Could you check a few things on this model? Use its own coordinates, in mm. A direction names the side the tool comes from. Coordinates: 2 decimals unless noted, no trailing zeros. Loops run counter-clockwise (first coordinate to the right, second up) from the corner with the lowest first, then second, coordinate; pieces in that order, holes last. Notation, with made-up numbers: (13.25, 69) - (47.25, 69) arc R35 ccw to (47.25, 101) - close; hole circle Ø5 at (65.5, -29.5). An arc over 180 degrees is marked (long way). One line per item, written item: value. Start each with the question number.
(1) I'm going to push flat-ended pins straight in: P1, Ø2, axis at y = -42.5, z = 1, coming from the +X side; P2, Ø1, axis at x = 9, y = -41, coming from the -Z side (3 decimals); P3, Ø12, axis at x = 7, y = -33, coming from the +Z side (3 decimals). Where does each tip first touch, or does it pass through?
(2) If we section it at D-D on y = -25: Write out the boundary of the cut face in (x, z) (3 decimals), then the cut area to 3 significant figures.
(3) If we section it at A-A on z = -1.5: Count the separate pieces of the cut face and the enclosed holes in it, then the cut area to 3 significant figures.
(4) If we section it at C-C on x = 0: Write out the boundary of the cut face in (y, z) (1 decimal), then the cut area to 3 significant figures.
(5) If we mould it in two halves opening along X, with no side actions, what happens to faces 1 (the face through (0, -48.26, 0)), 2 (the face through (5.556, -36, 0)), 3 (the face through (26.434, -18.68, 0.044)), 4 (the face through (-0.122, -27.624, 0.044))? For each: pulls with the +X half, pulls with the -X half, needs draft (parallel to the pull), parting line crosses it, or undercut.
(6) On a 3-axis mill with a long thin cutter (end or side, diameter ignored), from which of +Z, -Z, +X, -X, +Y, -Y can I reach the whole of each face in a straight line? I mean faces 5 (the face through (-9.45, -47.343, 0.044)), 6 (the face through (25.449, -25.404, 0.044)), 7 (the face through (10.319, -43, 0)). Say none if no direction works.
(7) If I drill on line 1 along Y through (x, z) = (0, 1.65); line 2 along X through (y, z) = (-34, -1); line 3 along Y through (x, z) = (1.5, -1.5), over which ranges is the centre line in solid material (lowest first)? Write a range as from..to.
```python
from build123d import *

# Parameters (mm, degrees)
SKETCH1_R           = 11.5062
BOSS_EXTRUDE2_DEPTH = 4.7625
BOSS_EXTRUDE3_DEPTH = 3.175
FILLET1_R           = 3.048
CHAMFER1_SIZE       = 0.889


with BuildPart() as part:
    # Sketch1 → Boss-Extrude2 (new body, symmetric)
    with BuildSketch(Plane.XY):
        with BuildLine():
            ThreePointArc((14.621497696, 1.322663433), (-4.556441994, 13.956234084), (-12.585193267, -7.559797873))
            ThreePointArc((-12.585193267, -7.559797873), (4.556441994, -13.956234084), (14.621497696, 1.322663433))
        make_face()
        Circle(SKETCH1_R, mode=Mode.SUBTRACT)
    extrude(amount=BOSS_EXTRUDE2_DEPTH, both=True)

    # Sketch1<4> → Boss-Extrude3 (add, symmetric)
    with BuildSketch(Plane.XY):
        with BuildLine():
            ThreePointArc((-12.585193267, -7.559797873), (-10.89585042, -11.492870345), (-10.31875, -15.734319794))
            Line((-10.31875, -15.734319794), (-10.31875, -48.26))
            Line((-10.31875, -48.26), (10.31875, -48.26))
            Line((10.31875, -48.26), (10.31875, -31.605996662))
            Line((10.31875, -31.605996662), (20.145719857, -45.051683354))
            Line((20.145719857, -45.051683354), (36.80750102, -32.874185469))
            Line((36.80750102, -32.874185469), (17.615185966, -6.614426983))
            ThreePointArc((17.615185966, -6.614426983), (15.578373329, -2.849545496), (14.621497696, 1.322663433))
            ThreePointArc((14.621497696, 1.322663433), (4.556441994, -13.956234084), (-12.585193267, -7.559797873))
        make_face()
        with BuildLine():
            ThreePointArc((5.55625, -37.94125), (0, -43.4975), (-5.55625, -37.94125))
            Line((-5.55625, -37.94125), (-5.55625, -33.17875))
            ThreePointArc((-5.55625, -33.17875), (0, -27.6225), (5.55625, -33.17875))
            Line((5.55625, -33.17875), (5.55625, -37.94125))
        make_face(mode=Mode.SUBTRACT)
        with BuildLine():
            ThreePointArc((26.873725655, -27.353486707), (25.666418619, -35.117907989), (17.901997337, -33.910600953))
            Line((17.901997337, -33.910600953), (15.091805517, -30.065574531))
            ThreePointArc((15.091805517, -30.065574531), (16.299112553, -22.301153249), (24.063533835, -23.508460285))
            Line((24.063533835, -23.508460285), (26.873725655, -27.353486707))
        make_face(mode=Mode.SUBTRACT)
    extrude(amount=BOSS_EXTRUDE3_DEPTH, both=True)

    # Fillet1
    fillet1_edges = [part.edges().sort_by_distance(p)[0] for p in [
        (-10.31875, -48.26, 0),
        (10.31875, -48.26, 0),
        (10.31875, -31.605996662, 0),
        (20.145719857, -45.051683354, 0),
        (36.80750102, -32.874185469, 0),
    ]]
    fillet(fillet1_edges, radius=FILLET1_R)

    # Chamfer1
    chamfer1_edges = [part.edges().sort_by_distance(p)[0] for p in [
        (-11.5062, 0, -4.7625),
        (-11.5062, 0, 4.7625),
    ]]
    chamfer(chamfer1_edges, length=CHAMFER1_SIZE)


solid = part.part
```
Values:
1. P1: stops at x = 25.01
1. P2: stops at z = -3.175
1. P3: stops at z = 3.175
2. outline: (-10.319, -3.175) - (14.317, -3.175) - (14.317, 3.175) - (-10.319, 3.175) - close; (25.154, -3.175) - (31.053, -3.175) - (31.053, 3.175) - (25.154, 3.175) - close
2. area: 194 mm2
3. separate pieces: 1
3. enclosed holes: 3
3. area: 1,300 mm2
4. outline: (-48.3, -3.2) - (-43.5, -3.2) - (-43.5, 3.2) - (-48.3, 3.2) - close; (-27.6, -3.2) - (-14.7, -3.2) - (-14.7, -4.8) - (-12.4, -4.8) - (-11.5, -3.9) - (-11.5, 3.9) - (-12.4, 4.8) - (-14.7, 4.8) - (-14.7, 3.2) - (-27.6, 3.2) - close; (11.5, -3.9) - (12.4, -4.8) - (14.7, -4.8) - (14.7, 4.8) - (12.4, 4.8) - (11.5, 3.9) - close
4. area: 171 mm2
5. face 1: needs draft
5. face 2: undercut
5. face 3: pulls with the +X half
5. face 4: undercut
6. face 5: +Z, -Z, -X, -Y
6. face 6: +Z, -Z
6. face 7: +Z, -Z, -Y
7. line 1: y = -48.26..-43.5, -27.62..-11.51, 11.51..14.68
7. line 2: x = -10.32..-5.56, 5.56..17.97, 26.81..35.02
7. line 3: y = -48.26..-43.29, -27.83..-11.41, 11.41..14.6
